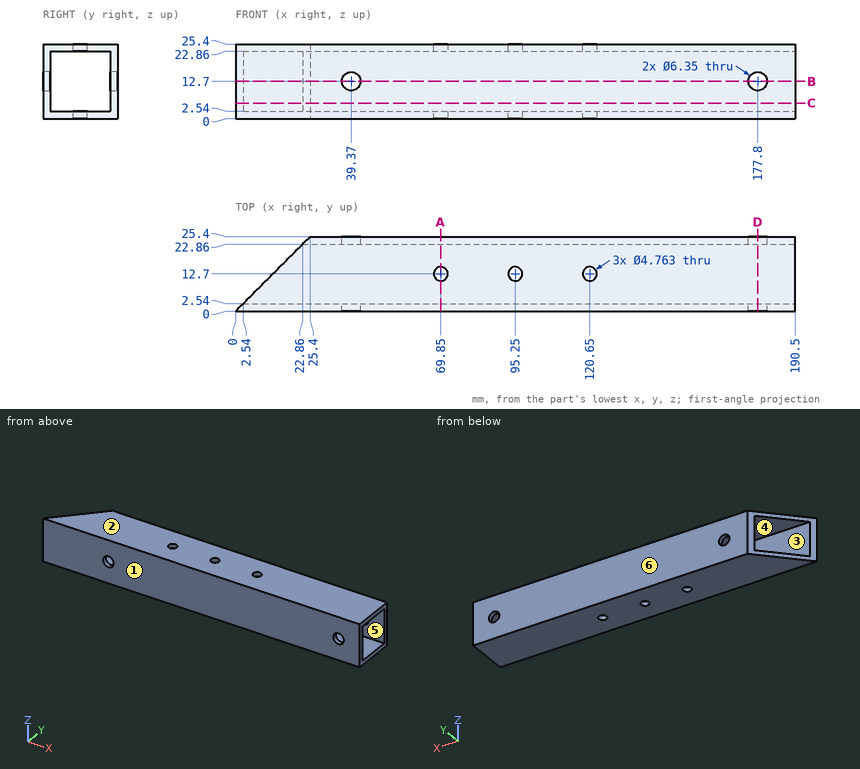
Answer from the drawing. Dimensions are ordinates in mm from the lowest x, y and z of the part. A direction names the side the tool comes from. Give positions to 0.01 mm unless a question says otherwise; leave off trailing zeros. Loops run counter-clockwise (first coordinate to the right, second up) from the corner with the lowest first, then second, coordinate; pieces in that order, holes last. Notation, with made-up numbers: (-21.5, 54.5) - (31.5, 54.5) arc R5 cw to (31.5, 61.5) - close; hole circle Ø10 at (-25.5, -27). An arc over 180 degrees is marked (long way). Answer as a JSON object with one key per item and string values.
1. A cutting plane is placed at D-D (x = 177.8). Write down the section's boundary in (y, z) (1 decimal).
Determined:
{"outline": "(0, 0) - (25.4, 0) - (25.4, 9.5) - (22.9, 9.5) - (22.9, 2.5) - (2.5, 2.5) - (2.5, 9.5) - (0, 9.5) - close; (0, 15.9) - (2.5, 15.9) - (2.5, 22.9) - (22.9, 22.9) - (22.9, 15.9) - (25.4, 15.9) - (25.4, 25.4) - (0, 25.4) - close"}
2. A cutting plane is placed at B-B (z = 12.7). Write down the section's boundary in (x, y) (1 decimal).
Determined:
{"outline": "(0, 0) - (36.2, 0) - (36.2, 2.5) - (2.5, 2.5) - close; (22.9, 22.9) - (36.2, 22.9) - (36.2, 25.4) - (25.4, 25.4) - close; (42.5, 0) - (174.6, 0) - (174.6, 2.5) - (42.5, 2.5) - close; (42.5, 22.9) - (174.6, 22.9) - (174.6, 25.4) - (42.5, 25.4) - close; (181, 0) - (190.5, 0) - (190.5, 2.5) - (181, 2.5) - close; (181, 22.9) - (190.5, 22.9) - (190.5, 25.4) - (181, 25.4) - close"}
3. A cutting plane is placed at C-C (z = 5.25). Write down the section's boundary in (x, y).
Determined:
{"outline": "(0, 0) - (190.5, 0) - (190.5, 2.54) - (2.54, 2.54) - close; (22.86, 22.86) - (190.5, 22.86) - (190.5, 25.4) - (25.4, 25.4) - close"}
4. A cutting plane is placed at A-A (x = 69.85). Write down the section's boundary in (y, z).
Determined:
{"outline": "(0, 0) - (10.32, 0) - (10.32, 2.54) - (2.54, 2.54) - (2.54, 22.86) - (10.32, 22.86) - (10.32, 25.4) - (0, 25.4) - close; (15.08, 0) - (25.4, 0) - (25.4, 25.4) - (15.08, 25.4) - (15.08, 22.86) - (22.86, 22.86) - (22.86, 2.54) - (15.08, 2.54) - close"}
5. Find the intervals of material crossed by L1, parallel to Z at x = 74, y = 12; L2, parallel to Y at x = 69.85, z = 24.2, in increasing order. Write a range as [from, to].
Determined:
{"L1": "[0, 2.54], [22.86, 25.4]", "L2": "[0, 10.32], [15.08, 25.4]"}
6. For the marked faces 5 and 6, determine the directions among +Z, -Z, +X, -X, +Y, -Y from which every point of the face is accessible in a straight line to the end or side of a thin tool.
Determined:
{"face 5": "+X, -X", "face 6": "+Z, -Z, +X, -X, +Y"}
7. Flat-ended cylindrical pins translate along their axes: pin 1 Ø6 at (x, y) = (120.65, 12.7) entering from -Z; pin 2 Ø12 at (y, z) = (14.5, 7.5) entering from -X (1 decimal). Find the tip coordinate at first contact, or state that the pin passes through.
Determined:
{"pin 1": "z = 0", "pin 2": "x = 11.1"}
8. For a pull along Z with two mould halves and no side action, classify the marked faces 1, 2, 3 and 4 as pulls with the +Z half, pulls with the -Z half, needs draft (parallel to the pull), parting line crosses it, or undercut.
Determined:
{"face 1": "needs draft", "face 2": "pulls with the +Z half", "face 3": "undercut", "face 4": "undercut"}
